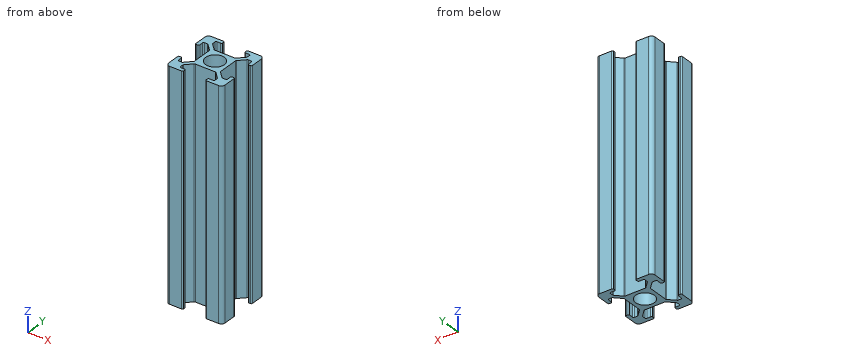
```python
from build123d import *

# Parameters (mm, degrees)
SKETCH1_R           = 2.5
BOSS_EXTRUDE1_DEPTH = 60


with BuildPart() as part:
    # Sketch1 → Boss-Extrude1 (new body)
    with BuildSketch(Plane.XY):
        with BuildLine():
            Line((0.997149379, -0.010991612), (4.197149379, -0.010991612))
            ThreePointArc((4.197149379, -0.010991612), (4.409281413, 0.076876353), (4.497149379, 0.289008388))
            Line((4.497149379, 0.289008388), (4.497149379, 0.689008388))
            ThreePointArc((4.497149379, 0.689008388), (4.409281413, 0.901140422), (4.197149379, 0.989008388))
            Line((4.197149379, 0.989008388), (3.197149379, 0.989008388))
            ThreePointArc((3.197149379, 0.989008388), (2.985017344, 1.076876353), (2.897149379, 1.289008388))
            Line((2.897149379, 1.289008388), (2.897149379, 2.057637538))
            ThreePointArc((2.897149379, 2.057637538), (2.920422177, 2.174637797), (2.9866975, 2.273825827))
            Line((2.9866975, 2.273825827), (4.61806835, 3.905196677))
            ThreePointArc((4.61806835, 3.905196677), (4.71725638, 3.971472), (4.834256639, 3.994744798))
            Line((4.834256639, 3.994744798), (10.171514939, 3.994744798))
            ThreePointArc((10.171514939, 3.994744798), (10.288515198, 3.971472), (10.387703228, 3.905196677))
            Line((10.387703228, 3.905196677), (12.019074078, 2.273825827))
            ThreePointArc((12.019074078, 2.273825827), (12.085349401, 2.174637797), (12.1086222, 2.057637538))
            Line((12.1086222, 2.057637538), (12.1086222, 1.289008388))
            ThreePointArc((12.1086222, 1.289008388), (12.020754234, 1.076876353), (11.8086222, 0.989008388))
            Line((11.8086222, 0.989008388), (10.797149379, 0.989008388))
            ThreePointArc((10.797149379, 0.989008388), (10.585017344, 0.901140422), (10.497149379, 0.689008388))
            Line((10.497149379, 0.689008388), (10.497149379, 0.289008388))
            ThreePointArc((10.497149379, 0.289008388), (10.585017344, 0.076876353), (10.797149379, -0.010991612))
            Line((10.797149379, -0.010991612), (13.997149379, -0.010991612))
            ThreePointArc((13.997149379, -0.010991612), (14.70425616, 0.281901607), (14.997149379, 0.989008388))
            Line((14.997149379, 0.989008388), (14.997149379, 4.189008388))
            ThreePointArc((14.997149379, 4.189008388), (14.909281413, 4.401140422), (14.697149379, 4.489008388))
            Line((14.697149379, 4.489008388), (14.305261888, 4.489008388))
            ThreePointArc((14.305261888, 4.489008388), (14.093129854, 4.401140422), (14.005261888, 4.189008388))
            Line((14.005261888, 4.189008388), (14.005261888, 3.189008388))
            ThreePointArc((14.005261888, 3.189008388), (13.917393922, 2.976876353), (13.705261888, 2.889008388))
            Line((13.705261888, 2.889008388), (12.936632738, 2.889008388))
            ThreePointArc((12.936632738, 2.889008388), (12.819632479, 2.912281186), (12.720444449, 2.978556509))
            Line((12.720444449, 2.978556509), (11.089073599, 4.609927359))
            ThreePointArc((11.089073599, 4.609927359), (11.006246661, 4.70520219), (10.969948855, 4.826115648))
            Line((10.969948855, 4.826115648), (10.969948855, 10.163373948))
            ThreePointArc((10.969948855, 10.163373948), (11.00546556, 10.284783861), (11.087867966, 10.380761184))
            Line((11.087867966, 10.380761184), (12.719238816, 12.012132034))
            ThreePointArc((12.719238816, 12.012132034), (12.81656582, 12.07716386), (12.93137085, 12.1))
            Line((12.93137085, 12.1), (13.7, 12.1))
            ThreePointArc((13.7, 12.1), (13.912132034, 12.012132034), (14, 11.8))
            Line((14, 11.8), (14, 10.8))
            ThreePointArc((14, 10.8), (14.087867966, 10.587867966), (14.3, 10.5))
            Line((14.3, 10.5), (14.697149379, 10.5))
            ThreePointArc((14.697149379, 10.5), (14.909281413, 10.587867966), (14.997149379, 10.8))
            Line((14.997149379, 10.8), (14.997149379, 13.989008388))
            ThreePointArc((14.997149379, 13.989008388), (14.70425616, 14.696115169), (13.997149379, 14.989008388))
            Line((13.997149379, 14.989008388), (10.797149379, 14.989008388))
            ThreePointArc((10.797149379, 14.989008388), (10.585017344, 14.901140422), (10.497149379, 14.689008388))
            Line((10.497149379, 14.689008388), (10.497149379, 14.289008388))
            ThreePointArc((10.497149379, 14.289008388), (10.585017344, 14.076876353), (10.797149379, 13.989008388))
            Line((10.797149379, 13.989008388), (11.798829534, 13.989008388))
            ThreePointArc((11.798829534, 13.989008388), (12.010961569, 13.901140422), (12.098829534, 13.689008388))
            Line((12.098829534, 13.689008388), (12.098829534, 12.916322983))
            ThreePointArc((12.098829534, 12.916322983), (12.075993394, 12.801517953), (12.010961569, 12.704190949))
            Line((12.010961569, 12.704190949), (10.379590719, 11.072820099))
            ThreePointArc((10.379590719, 11.072820099), (10.282263714, 11.007788273), (10.167458684, 10.984952133))
            Line((10.167458684, 10.984952133), (4.830200384, 10.984952133))
            ThreePointArc((4.830200384, 10.984952133), (4.715395355, 11.007788273), (4.61806835, 11.072820099))
            Line((4.61806835, 11.072820099), (2.9866975, 12.704190949))
            ThreePointArc((2.9866975, 12.704190949), (2.920422177, 12.803378979), (2.897149379, 12.920379238))
            Line((2.897149379, 12.920379238), (2.897149379, 13.689008388))
            ThreePointArc((2.897149379, 13.689008388), (2.985017344, 13.901140422), (3.197149379, 13.989008388))
            Line((3.197149379, 13.989008388), (4.197149379, 13.989008388))
            ThreePointArc((4.197149379, 13.989008388), (4.409281413, 14.076876353), (4.497149379, 14.289008388))
            Line((4.497149379, 14.289008388), (4.497149379, 14.689008388))
            ThreePointArc((4.497149379, 14.689008388), (4.409281413, 14.901140422), (4.197149379, 14.989008388))
            Line((4.197149379, 14.989008388), (0.997149379, 14.989008388))
            ThreePointArc((0.997149379, 14.989008388), (0.290042597, 14.696115169), (-0.002850621, 13.989008388))
            Line((-0.002850621, 13.989008388), (-0.002850621, 10.789008388))
            ThreePointArc((-0.002850621, 10.789008388), (0.085017344, 10.576876353), (0.297149379, 10.489008388))
            Line((0.297149379, 10.489008388), (0.697149379, 10.489008388))
            ThreePointArc((0.697149379, 10.489008388), (0.909281413, 10.576876353), (0.997149379, 10.789008388))
            Line((0.997149379, 10.789008388), (0.997149379, 11.790199043))
            ThreePointArc((0.997149379, 11.790199043), (1.085017344, 12.002331078), (1.297149379, 12.090199043))
            Line((1.297149379, 12.090199043), (2.057928823, 12.090199043))
            ThreePointArc((2.057928823, 12.090199043), (2.174143192, 12.067250491), (2.272911478, 12.001849869))
            Line((2.272911478, 12.001849869), (3.912132034, 10.380761184))
            ThreePointArc((3.912132034, 10.380761184), (3.97928656, 10.281159192), (4.002885789, 10.163373948))
            Line((4.002885789, 10.163373948), (4.002885789, 4.826115648))
            ThreePointArc((4.002885789, 4.826115648), (3.979612991, 4.709115389), (3.913337668, 4.609927359))
            Line((3.913337668, 4.609927359), (2.281966818, 2.978556509))
            ThreePointArc((2.281966818, 2.978556509), (2.182778788, 2.912281186), (2.065778529, 2.889008388))
            Line((2.065778529, 2.889008388), (1.297149379, 2.889008388))
            ThreePointArc((1.297149379, 2.889008388), (1.085017344, 2.976876353), (0.997149379, 3.189008388))
            Line((0.997149379, 3.189008388), (0.997149379, 4.189008388))
            ThreePointArc((0.997149379, 4.189008388), (0.909281413, 4.401140422), (0.697149379, 4.489008388))
            Line((0.697149379, 4.489008388), (0.297149379, 4.489008388))
            ThreePointArc((0.297149379, 4.489008388), (0.085017344, 4.401140422), (-0.002850621, 4.189008388))
            Line((-0.002850621, 4.189008388), (-0.002850621, 0.989008388))
            ThreePointArc((-0.002850621, 0.989008388), (0.290042597, 0.281901607), (0.997149379, -0.010991612))
        make_face()
        with Locations((7.5, 7.5)):
            Circle(SKETCH1_R, mode=Mode.SUBTRACT)
    extrude(amount=BOSS_EXTRUDE1_DEPTH)


solid = part.part
```
Could you check a few things on this model? Use its own coordinates, in mm. Coordinates: 2 decimals unless noted, no trailing zeros. Write each loop counter-clockwise with the first axis right and the second up, starting at its lowest first coordinate (ties: lowest second). Pieces come first, ordered by that corner, then holes. Notation, with made-up numbers: (-1, 22.25) -> (20, 22.25) arc R22 cw to (20, 44.25) -> close; hole circle Ø8 at (23, 62). An arc over 180 degrees is marked (long way). One line per question, with ' | ' between items. Start each with the question number.
1. Please list where these lines run through material, in increasing order: line 1 along Y through (x, z) = (1.75, 44); line 2 along Y through (x, z) = (7.5, 44.5); line 3 along X through (y, z) = (12, 53).
2. If we section it at A-A (x = 7.5): Please give me the cut outline in (y, z).
3. If we section it at B-B (y = 7.5): Please give me the cut outline in (x, z).
4. Will these pins go through, and if not, where does the flat tip stop? P1, Ø2, axis at x = 13, y = 6, coming from the +Z side; P2, Ø1.6, axis at x = 7, z = 25.5, coming from the +Y side; P3, Ø1.5, axis at y = 9, z = 51.5, coming from the +X side.
Return value:
1) line 1: y = -0.01 to 2.89, 12.09 to 14.99 | line 2: y = 3.99 to 5, 10 to 10.98 | line 3: x = 0 to 1.08, 2.27 to 3.69, 11.31 to 12.71, 13.92 to 15
2) outline: (3.99, 0) -> (5, 0) -> (5, 60) -> (3.99, 60) -> close; (10, 0) -> (10.98, 0) -> (10.98, 60) -> (10, 60) -> close
3) outline: (4, 0) -> (5, 0) -> (5, 60) -> (4, 60) -> close; (10, 0) -> (10.97, 0) -> (10.97, 60) -> (10, 60) -> close
4) P1: passes through | P2: stops at y = 10.98 | P3: stops at x = 10.97
